Job drawing, mm, ordinate dimensions from the low corner. One solid piece. Coordinates: 2 decimals unless noted, no trailing zeros. Order: outer loops, then holes, each group sorted by start corner. A loop starts at its lowest first (then second) coordinate and runs counter-clockwise, first axis right, second up. Notation, with made-up numbers: (62.25, 49.25) - (113.25, 49.25) arc R11 ccw to (113.25, 62.25) - close; hole circle Ø7 at (51.5, 5). An arc over 180 degrees is marked (long way). Use a Markdown table: item, result. Add a question column.
1) Drop a flat-ended pin along its axis: P1, Ø2, axis at x = 177.5, z = 4, coming from the -Y side. Give the stop position or say it passes through.
2) Wall check: L1, parallel to Y at x = 25.4, z = 6.5; L2, parallel to Y at x = 103, z = 9.5. Give the ranges that are in metal, low to high. Write a range as [from, to].
3) Saw through at B-B on x = 177.8. List the corners of the cut face in (y, z), then the cut area to 3 significant figures.
4) Two-plate mould, pull along Z, no slides. Class the marked faces 1 and 2: +Z half, -Z half, draft (parallel to the pull), parting line (faces both ways), or undercut.
5) Saw through at A-A on y = 50.8. Count the separate pieces of the cut face and the enclosed holes in it, then the cut area to 3 significant figures.
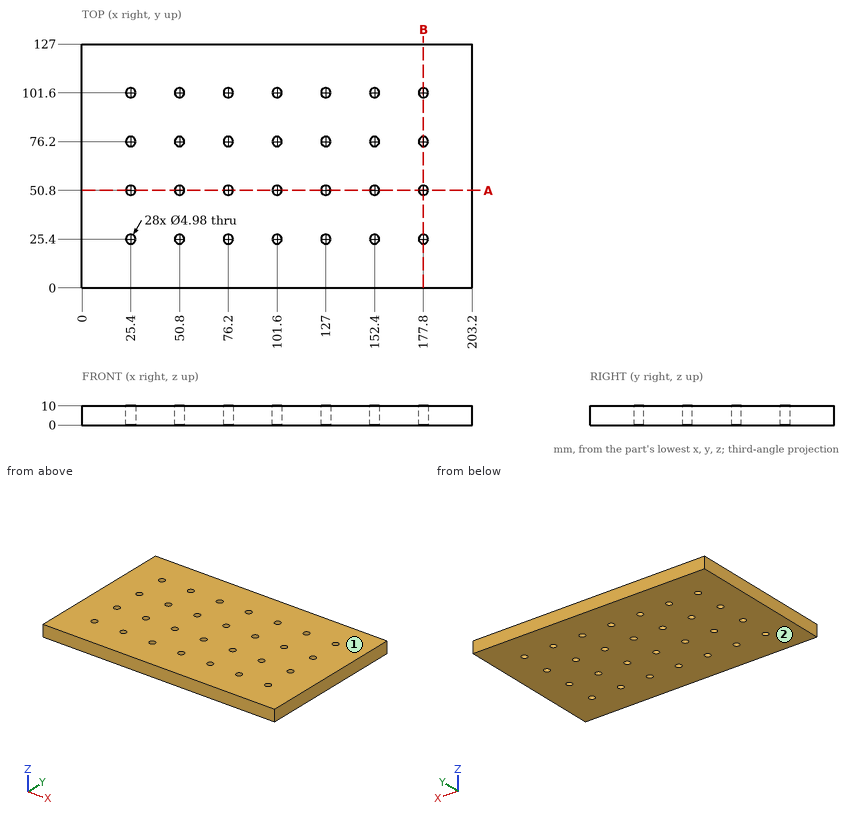
Results are:
| question | item | result |
|---|---|---|
| 1 | P1 | y = 0 |
| 2 | L1 | [0, 22.91], [27.89, 48.31], [53.29, 73.71], [78.69, 99.11], [104.09, 127] |
| 2 | L2 | [0, 23.34], [27.46, 48.74], [52.86, 74.14], [78.26, 99.54], [103.66, 127] |
| 3 | outline | (0, 0) - (22.91, 0) - (22.91, 10) - (0, 10) - close; (27.89, 0) - (48.31, 0) - (48.31, 10) - (27.89, 10) - close; (53.29, 0) - (73.71, 0) - (73.71, 10) - (53.29, 10) - close; (78.69, 0) - (99.11, 0) - (99.11, 10) - (78.69, 10) - close; (104.09, 0) - (127, 0) - (127, 10) - (104.09, 10) - close |
| 3 | area | 1,070 mm2 |
| 4 | face 1 | +Z half |
| 4 | face 2 | -Z half |
| 5 | separate pieces | 8 |
| 5 | enclosed holes | 0 |
| 5 | area | 1,680 mm2 |
